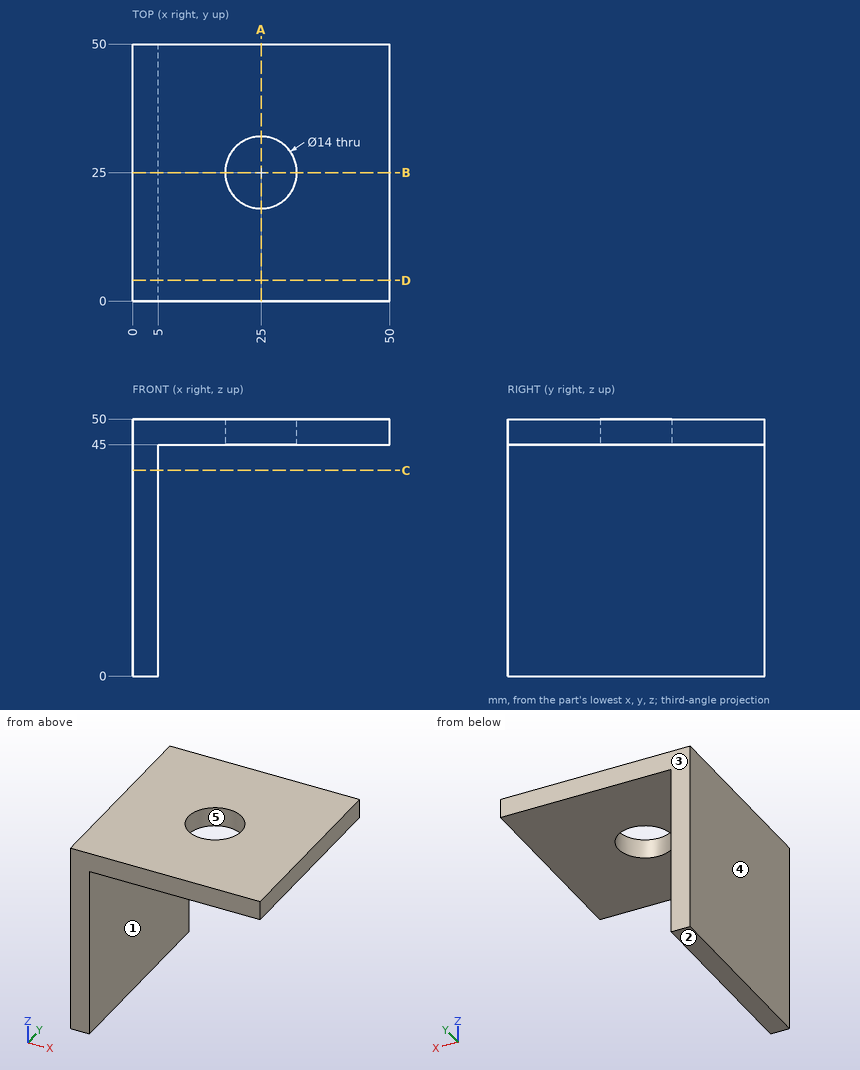
Study the drawing (mm; zero at the part's minimum x, y, z) and answer. A direction names the side the tool comes from. Give positions to 0.01 mm unless a question says otherwise; leave off trailing zeros. Loops run counter-clockwise (first coordinate to the right, second up) from the corner with the lowest first, then second, coordinate; pieces in that order, holes last. Notation, with made-up numbers: (-32.75, 1) - (-19.75, 1) arc R9 ccw to (-19.75, 7) - close; hole circle Ø10 at (-30.75, 89). An arc over 180 degrees is marked (long way). Use CSV: the item, a comma, the result in double quotes. Start each with the question number.
(1) Each of these flat-tipped pins is pushed along its axis until it touches: pin 1 (22.5 mm diameter, centred on x = 32, y = 32.5, fed in from -Z); pin 2 (5 mm diameter, centred on y = 33.5, z = 6, fed in from +X). Where does it stop, or does it pass through?
(2) Find section A-A, the plane x = 25. Determine the outline of the cut face in (y, z).
(3) A tool of negligible diameter and unlimited length cuts with its end or side. For the marked faces 1 and 2, from which of +Z, -Z, +X, -X, +Y, -Y can it reach the whole face along a straight path? Write none if from no direction.
(4) Find the intervals of material crossed by L1, parallel to Y at x = 25, z = 46.35; L2, parallel to Z at x = 31.5, y = 7; L3, parallel to X at y = 26.5, z = 33, in increasing order.
(5) Find section C-C, the plane z = 40. Determine the outline of the cut face in (x, y), plus the area to 3 significant figures.
(6) Find section B-B, the plane y = 25. Determine the outline of the cut face in (x, z).
(7) Determine the mould class of the marked faces 3, 4 and 5 for opening direction Y: released by +Y, released by -Y, zero draft, split by the parting line, or undercut.
(8) Find section D-D, the plane y = 4. Determine the outline of the cut face in (x, z), plus the area to 3 significant figures.
Results found:
1,pin 1,"z = 45"
1,pin 2,"x = 5"
2,outline,"(0, 45) - (18, 45) - (18, 50) - (0, 50) - close; (32, 45) - (50, 45) - (50, 50) - (32, 50) - close"
3,face 1,"-Z, +X, +Y, -Y"
3,face 2,"-Z, +X, -X, +Y, -Y"
4,L1,"0 to 18, 32 to 50"
4,L2,"45 to 50"
4,L3,"0 to 5"
5,outline,"(0, 0) - (5, 0) - (5, 50) - (0, 50) - close"
5,area,"250 mm^2"
6,outline,"(0, 0) - (5, 0) - (5, 45) - (18, 45) - (18, 50) - (0, 50) - close; (32, 45) - (50, 45) - (50, 50) - (32, 50) - close"
7,face 3,"released by +Y"
7,face 4,"zero draft"
7,face 5,"undercut"
8,outline,"(0, 0) - (5, 0) - (5, 45) - (50, 45) - (50, 50) - (0, 50) - close"
8,area,"475 mm^2"
